```python
from build123d import *

# Parameters (mm, degrees)
SKETCH2_W                  = 80
SKETCH2_H                  = 60
SKETCH2_W_2                = 40
SKETCH2_H_2                = 24
LID_FRAME_DEPTH            = 2.4
SNAP_LEFT_START            = -18
SKETCH3_W                  = 1.2
SKETCH3_H                  = 8
SNAP_LEFT_DEPTH            = 18
SNAP_RIGHT_START           = -18
SKETCH4_W                  = 1.2
SKETCH4_H                  = 8
SNAP_RIGHT_DEPTH           = 18
HOOK_LEFT_START            = -17
SKETCH5_W                  = 0.8
SKETCH5_H                  = 8
HOOK_LEFT_DEPTH            = 1.5
HOOK_RIGHT_START           = -17
SKETCH6_W                  = 0.8
SKETCH6_H                  = 8
HOOK_RIGHT_DEPTH           = 1.5
SKETCH8_R                  = 2.2
SHAFT_CLEARANCE_D4P4_DEPTH = 54.141321022


with BuildPart() as part:
    # Sketch2 → Lid_frame (new body)
    with BuildSketch(Plane.XY):
        Rectangle(SKETCH2_W, SKETCH2_H)
        Rectangle(SKETCH2_W_2, SKETCH2_H_2, mode=Mode.SUBTRACT)
    extrude(amount=LID_FRAME_DEPTH)

    # Sketch3 → Snap_left (add)
    with BuildSketch(Plane.XY.offset(SNAP_LEFT_START)):
        with Locations((-35.9, 0)):
            Rectangle(SKETCH3_W, SKETCH3_H)
    extrude(amount=SNAP_LEFT_DEPTH)

    # Sketch4 → Snap_right (add)
    with BuildSketch(Plane.XY.offset(SNAP_RIGHT_START)):
        with Locations((35.9, 0)):
            Rectangle(SKETCH4_W, SKETCH4_H)
    extrude(amount=SNAP_RIGHT_DEPTH)

    # Sketch5 → Hook_left (add)
    with BuildSketch(Plane.XY.offset(HOOK_LEFT_START)):
        with Locations((-36.9, 0)):
            Rectangle(SKETCH5_W, SKETCH5_H)
    extrude(amount=HOOK_LEFT_DEPTH)

    # Sketch6 → Hook_right (add)
    with BuildSketch(Plane.XY.offset(HOOK_RIGHT_START)):
        with Locations((36.9, 0)):
            Rectangle(SKETCH6_W, SKETCH6_H)
    extrude(amount=HOOK_RIGHT_DEPTH)

    # Sketch8 → Shaft_clearance_D4p4 (cut, through all)
    with BuildSketch(Plane.XY):
        with Locations((0, 20.5)):
            Circle(SKETCH8_R)
    extrude(amount=SHAFT_CLEARANCE_D4P4_DEPTH, mode=Mode.SUBTRACT)


solid = part.part
```
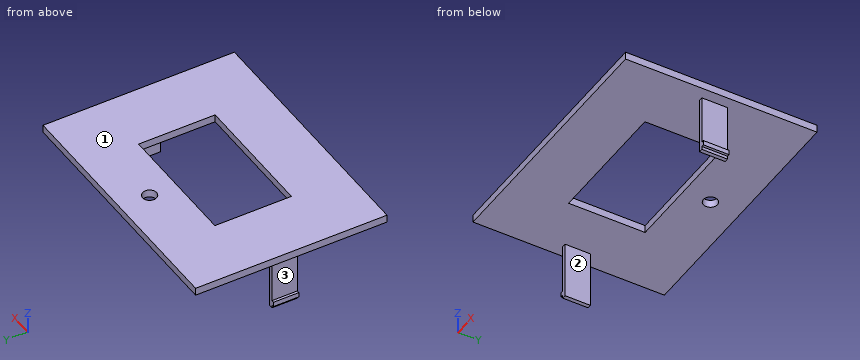
Can you work these out from the model? Positions are in its coordinate system, mm. Face numbers are marked on the shaded views. Give positions to 0.01 mm unless a question says otherwise; leave off trailing zeros. Order: outer loops, then holes, each group sorted by start corner. A loop starts at its lowest first (then second) coordinate and runs counter-clockwise, first axis right, second up. Notation, with made-up numbers: (-33.5, 13) - (-9.5, 13) arc R13 cw to (-9.5, 37) - close; hole circle Ø2 at (-13.5, -3). An arc over 180 degrees is marked (long way). Use a Markdown table: item, result. Add a question column.
Q1. If we section it at D-D on x = -21: Write out the boundary of the cut face in (y, z).
Q2. If we section it at B-B on x = 0: Write out the boundary of the cut face in (y, z).
Q3. If we section it at C-C on y = 10: Write out the boundary of the cut face in (x, z).
Q4. I'm going to push flat-ended pins straight in: pin 1 (0.6 mm diameter, centred on x = 36.5, z = -4.5, fed in from -Y); pin 2 (9 mm diameter, centred on y = 0.5, z = -7.5, fed in from +X); pin 3 (4 mm diameter, centred on y = 0, z = -8.5, fed in from -X). Where does each tip first touch, or does it pass through?
Q5. If we mould it in two halves opening along Z, with no side actions, what happens to the marked faces 1, 2 and 3? For each: released by +Z, released by -Z, zero draft, split by the parting line, or undercut.
Q6. Please list where these lines run through material, in increasing order: line 1 along X through (y, z) = (20.5, 0.55); line 2 along Y through (x, z) = (0, 0.9); line 3 along X through (y, z) = (6, 0.5).
Q7. If we section it at A-A on z = -1.5: Write out the boundary of the cut face in (x, y).
Answers follow:
| question | item | result |
|---|---|---|
| 1 | outline | (-30, 0) - (30, 0) - (30, 2.4) - (-30, 2.4) - close |
| 2 | outline | (-30, 0) - (-12, 0) - (-12, 2.4) - (-30, 2.4) - close; (12, 0) - (18.3, 0) - (18.3, 2.4) - (12, 2.4) - close; (22.7, 0) - (30, 0) - (30, 2.4) - (22.7, 2.4) - close |
| 3 | outline | (-40, 0) - (-20, 0) - (-20, 2.4) - (-40, 2.4) - close; (20, 0) - (40, 0) - (40, 2.4) - (20, 2.4) - close |
| 4 | pin 1 | stops at y = -4 |
| 4 | pin 2 | stops at x = 36.5 |
| 4 | pin 3 | stops at x = -36.5 |
| 5 | face 1 | released by +Z |
| 5 | face 2 | zero draft |
| 5 | face 3 | undercut |
| 6 | line 1 | x = -40 to -2.2, 2.2 to 40 |
| 6 | line 2 | y = -30 to -12, 12 to 18.3, 22.7 to 30 |
| 6 | line 3 | x = -40 to -20, 20 to 40 |
| 7 | outline | (-36.5, -4) - (-35.3, -4) - (-35.3, 4) - (-36.5, 4) - close; (35.3, -4) - (36.5, -4) - (36.5, 4) - (35.3, 4) - close |
